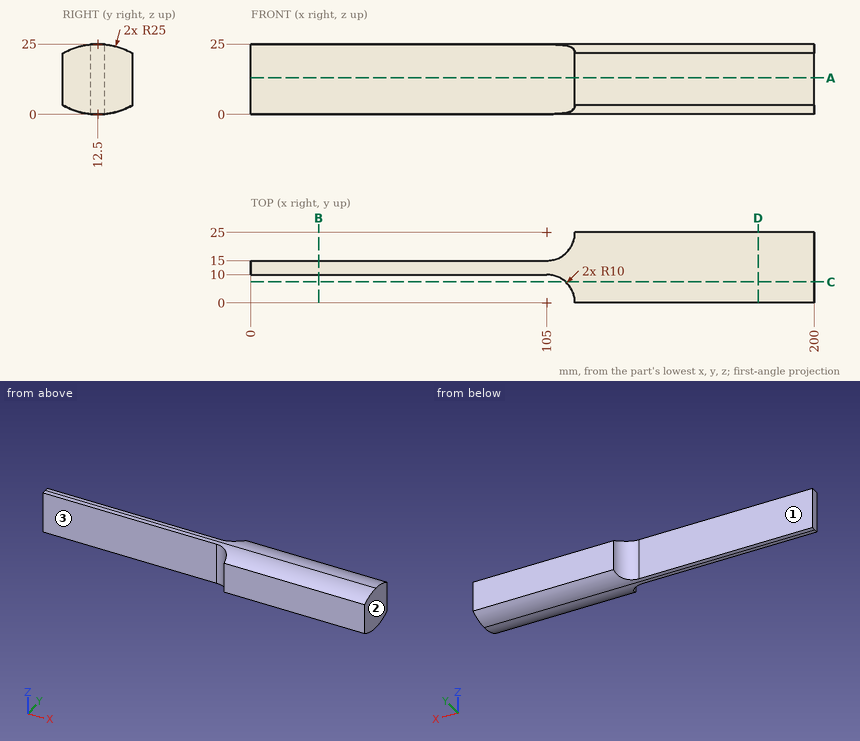
Input: dimensioned drawing with shaded views. Units: mm. Origin: part minimum x, y, z. A direction names the side the tool comes from. Give positions to 0.01 mm unless a question says otherwise; leave off trailing zeros. Write each loop counter-clockwise with the first axis right and the second up, starting at its lowest first coordinate (ties: lowest second). Pieces come first, ordered by that corner, then holes. Notation, with made-up numbers: (-36.5, -3) - (1.5, -3) arc R16 ccw to (1.5, 13) - close; hole circle Ø6 at (44, 84.5). An arc over 180 degrees is marked (long way). One line per item, written item: value. Start each with the question number.
Q1. First-contact query: pin 1 Ø4 at (y, z) = (16, 9) entering from -X; pin 2 Ø8 at (x, z) = (88, 20) entering from +Y; pin 3 Ø8 at (x, z) = (104.5, 6.5) entering from +Y; pin 4 Ø10 at (x, z) = (84.5, 19.5) entering from -Y. Flat tips, straight axial feed; report the tip coordinate or a pass-through.
Q2. Section query D-D, the plane x = 180. Return the cut outline in (y, z).
Q3. Section query B-B, the plane x = 24. Return the cut outline in (y, z).
Q4. Material intervals for probe 1 along Z at (x, y) = (128.5, 14.75); probe 2 along Y at (x, z) = (98.5, 17); probe 3 along Z at (x, y) = (140.5, 13.25), sorted ascending. Write a range as from..to.
Q5. Section query C-C, the plane y = 7.5. Return the cut outline in (x, z).
Q6. Set-up query: the marked faces 1, 2 and 3. Return all of +Z, -Z, +X, -X, +Y, -Y with unobstructed straight access to the full face (end or side cutting, diameter ignored); none if empty.
Q7. Section query A-A, the plane z = 13. Return the cut outline in (x, y).
Answer:
1. pin 1: stops at x = 0
1. pin 2: stops at y = 15
1. pin 3: stops at y = 15.63
1. pin 4: stops at y = 10
2. outline: (0, 3.35) arc R25 ccw to (12.5, 0) arc R25 ccw to (25, 3.35) - (25, 21.65) arc R25 ccw to (12.5, 25) arc R25 ccw to (0, 21.65) - close
3. outline: (10, 0.13) arc R25 ccw to (12.5, 0) arc R25 ccw to (15, 0.13) - (15, 24.87) arc R25 ccw to (12.5, 25) arc R25 ccw to (10, 24.87) - close
4. probe 1: z = 0.1..24.9
4. probe 2: y = 10..15
4. probe 3: z = 0.01..24.99
5. outline: (111.61, 0.51) - (200, 0.51) - (200, 24.49) - (111.61, 24.49) - close
6. face 1: +Z, -Z, -X, +Y
6. face 2: +Z, -Z, +X, +Y, -Y
6. face 3: +Z, -Z, -X, -Y
7. outline: (0, 10) - (105, 10) arc R10 cw to (115, 0) - (200, 0) - (200, 25) - (115, 25) arc R10 cw to (105, 15) - (0, 15) - close
